Input: part model. Units: mm. Frame: model coordinates. A direction names the side the tool comes from. Give positions to 0.01 mm unless a question says otherwise; leave off trailing zeros. Order: outer loops, then holes, each group sorted by start corner. A loop starts at its lowest first (then second) coordinate and runs counter-clockwise, first axis right, second up. Notation, with made-up numbers: (29.5, -15) - (53.5, -15) arc R16 ccw to (53.5, -5) - close; hole circle Ø1 at (20.25, -23.75). An arc over 180 degrees is marked (long way). Use a Markdown table: item, result.
from build123d import *

# Parameters (mm, degrees)
SKETCH_3_R               = 3
EXTRUDE_6_DEPTH          = 0.001
EXTRUDE_6_2_DEPTH        = 0.001
EXTRUDE_6_3_DEPTH        = 0.001
EXTRUDE_6_4_DEPTH        = 0.001
SKETCH_11_R              = 2.25
CUT_EXTRUDE_2_DEPTH      = 1
CUT_EXTRUDE_2_DEPTH_BACK = 1.001
EXTRUDE_7_DEPTH          = 3
SKETCH_14_R              = 2.25
SKETCH_14_R_2            = 10
CUT_EXTRUDE_3_DEPTH      = 3
SKETCH_15_R              = 10
SKETCH_15_R_2            = 1.5
CUT_EXTRUDE_4_DEPTH      = 3
SKETCH_16_R              = 1.5
CUT_EXTRUDE_5_DEPTH      = 10
SKETCH_17_R              = 7.5
SKETCH_17_R_2            = 5.5
EXTRUDE_8_DEPTH          = 7
FILLET_1_R               = 10


with BuildPart() as part:
    # Sketch 3 → Extrude 6 (new body)
    with BuildSketch(Plane.XY):
        with Locations((60.266478541, 16.532501821)):
            Circle(SKETCH_3_R)
    extrude(amount=EXTRUDE_6_DEPTH)


with BuildPart() as body_2:
    # Sketch 3 → Extrude 6 2 (new body)
    with BuildSketch(Plane.XY):
        with Locations((60.266478541, 6.532501821)):
            Circle(SKETCH_3_R)
    extrude(amount=EXTRUDE_6_2_DEPTH)


with BuildPart() as body_3:
    # Sketch 3 → Extrude 6 3 (new body)
    with BuildSketch(Plane.XY):
        with Locations((10.766478541, 6.532501821)):
            Circle(SKETCH_3_R)
    extrude(amount=EXTRUDE_6_3_DEPTH)


with BuildPart() as body_4:
    # Sketch 3 → Extrude 6 4 (new body)
    with BuildSketch(Plane.XY):
        with Locations((10.766478541, 16.532501821)):
            Circle(SKETCH_3_R)
    extrude(amount=EXTRUDE_6_4_DEPTH)


with BuildPart() as cut_extrude_2_tool:
    # Sketch 11 → Cut-Extrude 2 (new body, two sides)
    with BuildSketch(Plane.XY.offset(0.001)) as cut_extrude_2_sk:
        with Locations((10.766478541, 16.532501821)):
            Circle(SKETCH_11_R)
        with Locations((10.766478541, 6.532501821)):
            Circle(SKETCH_11_R)
        with Locations((60.266478541, 16.532501821)):
            Circle(SKETCH_11_R)
        with Locations((60.266478541, 6.532501821)):
            Circle(SKETCH_11_R)
    extrude(amount=CUT_EXTRUDE_2_DEPTH)
    extrude(cut_extrude_2_sk.sketch, amount=-CUT_EXTRUDE_2_DEPTH_BACK)


with BuildPart() as part_1:
    add(part.part)

    # Cut-Extrude 2: cut by cut_extrude_2_tool
    add(cut_extrude_2_tool.part, mode=Mode.SUBTRACT)



with BuildPart() as body_2_1:
    add(body_2.part)

    # Cut-Extrude 2: cut by cut_extrude_2_tool
    add(cut_extrude_2_tool.part, mode=Mode.SUBTRACT)


with BuildPart() as body_3_1:
    add(body_3.part)

    # Cut-Extrude 2: cut by cut_extrude_2_tool
    add(cut_extrude_2_tool.part, mode=Mode.SUBTRACT)


with BuildPart() as body_4_1:
    add(body_4.part)

    # Cut-Extrude 2: cut by cut_extrude_2_tool
    add(cut_extrude_2_tool.part, mode=Mode.SUBTRACT)


with BuildPart() as part_2:
    add(part_1.part)

    add(body_2_1.part)  # Extrude 7 merges body 2

    add(body_3_1.part)  # Extrude 7 merges body 3

    add(body_4_1.part)  # Extrude 7 merges body 4
    # Sketch 12 → Extrude 7 (add)
    with BuildSketch(Plane.XY.offset(0.001)):
        Polygon((5.516478541, 26.532501821), (65.516478541, 26.532501821), (65.516478541, -28.467498179), (5.516478541, -28.467498179), (5.516478541, 1.532501821), align=None)
    extrude(amount=EXTRUDE_7_DEPTH)

    # Sketch 14 → Cut-Extrude 3 (cut)
    with BuildSketch(Plane(origin=(0, 0, 0.001), x_dir=(-1, 0, 0), z_dir=(0, 0, -1))):
        with Locations((-60.266478541, 6.532501821)):
            Circle(SKETCH_14_R)
        with Locations((-60.266478541, 16.532501821)):
            Circle(SKETCH_14_R)
        with Locations((-10.766478541, 6.532501821)):
            Circle(SKETCH_14_R)
        with Locations((-10.766478541, 16.532501821)):
            Circle(SKETCH_14_R)
        with Locations((-45.516478541, 11.532501821)):
            Circle(SKETCH_14_R_2)
    extrude(amount=-CUT_EXTRUDE_3_DEPTH, mode=Mode.SUBTRACT)

    # Sketch 15 → Cut-Extrude 4 (cut)
    with BuildSketch(Plane(origin=(0, 0, 0.001), x_dir=(-1, 0, 0), z_dir=(0, 0, -1))):
        with Locations((-45.516478541, 11.532501821)):
            Circle(SKETCH_15_R)
        with Locations((-45.516478541, -13.567498179)):
            Circle(SKETCH_15_R_2)
    extrude(amount=-CUT_EXTRUDE_4_DEPTH, mode=Mode.SUBTRACT)

    # Sketch 16 → Cut-Extrude 5 (cut)
    with BuildSketch(Plane.XY.offset(3.001)):
        with Locations((10.016478541, -8.467498179)):
            Circle(SKETCH_16_R)
        with Locations((25.016478541, -8.467498179)):
            Circle(SKETCH_16_R)
    extrude(amount=-CUT_EXTRUDE_5_DEPTH, mode=Mode.SUBTRACT)

    # Sketch 17 → Extrude 8 (add)
    with BuildSketch(Plane.XY.offset(3.001)):
        with Locations((45.516478541, -13.567498179)):
            Circle(SKETCH_17_R)
        with Locations((45.516478541, -13.567498179)):
            Circle(SKETCH_17_R_2, mode=Mode.SUBTRACT)
    extrude(amount=-EXTRUDE_8_DEPTH)

    # Fillet 1
    fillet_1_edges = [part_2.edges().sort_by_distance(p)[0] for p in [
        (5.516478541, 26.532501821, 1.501),
        (5.516478541, -28.467498179, 1.501),
        (65.516478541, -28.467498179, 1.501),
        (65.516478541, 26.532501821, 1.501),
    ]]
    fillet(fillet_1_edges, radius=FILLET_1_R)


solid = part_2.part
1. Material intervals for line 1 along X through (y, z) = (6.5, 0.5); line 2 along Z through (x, y) = (28, 15); line 3 along X through (y, z) = (15, 1.5), sorted ascending.
Response:
| item | result |
|---|---|
| line 1 | x = 5.52 to 8.52, 13.02 to 36.88, 54.16 to 58.02, 62.52 to 65.52 |
| line 2 | z = 0 to 3 |
| line 3 | x = 5.52 to 9.12, 12.41 to 36.14, 54.9 to 58.62, 61.91 to 65.52 |
2. Mould query, pull axis Y, two halves, no side actions, for faces 3 (the face through (35.98, 14.54, 1.48)), 4 (the face through (36, -28.467, 1)), 5 (the face through (11, 19, 0)). Classes: pulls with the +Y half, pulls with the -Y half, needs draft (parallel to the pull), parting line crosses it, or undercut.
Response:
| item | result |
|---|---|
| face 3 | undercut |
| face 4 | pulls with the -Y half |
| face 5 | needs draft |
3. Section query B-B (x = 59). State how many separate pieces and enclosed holes the cut face has, then the cut area to 3 significant figures.
Response:
| item | result |
|---|---|
| separate pieces | 3 |
| enclosed holes | 0 |
| area | 139 mm^2 |
4. Section query A-A (x = 39). Return loops of the section in (y, z).
Response:
| item | result |
|---|---|
| outline | (-28.47, 0) - (-17.28, 0) - (-17.28, -4) - (-9.85, -4) - (-9.85, 0) - (3.95, 0) - (3.95, 3) - (-28.47, 3) - close; (19.12, 0) - (26.53, 0) - (26.53, 3) - (19.12, 3) - close |
5. Set-up query: faces 1 (the face through (40.02, -13.33, -1.97)), 2 (the face through (5.516, -1, 1)). Return all of +Z, -Z, +X, -X, +Y, -Y with unobstructed straight access to the full face (end or side cutting, diameter ignored); none if empty.
Response:
| item | result |
|---|---|
| face 1 | -Z |
| face 2 | +Z, -Z, -X, +Y, -Y |
6. Pin query (flat end, axial travel): pin 1 (1 mm diameter, centred on y = 0, z = -2, fed in from +X); pin 2 (3.5 mm diameter, centred on x = 25.02, y = -8.47, fed in from -Z). Return the tip coordinate at first contact, or that it passes through.
Response:
| item | result |
|---|---|
| pin 1 | passes through |
| pin 2 | stops at z = 0 |
